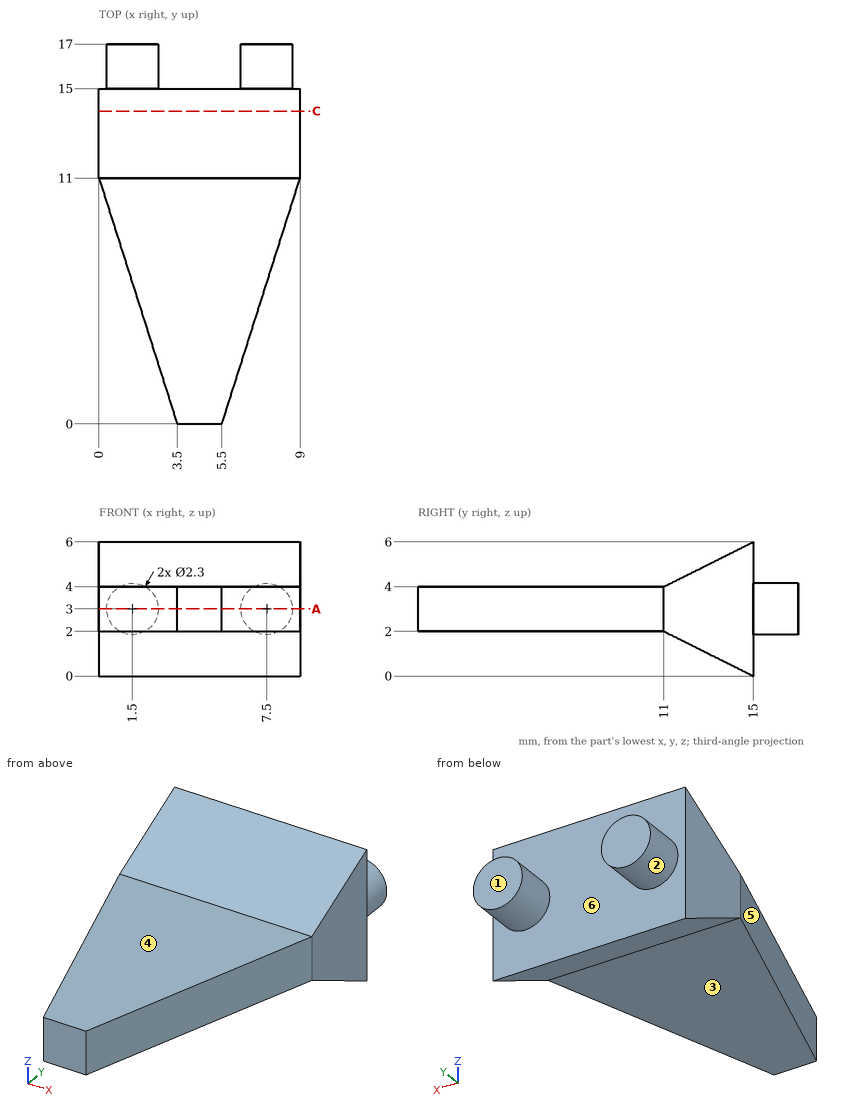
Study the drawing (mm; zero at the part's minimum x, y, z) and answer. A direction names the side the tool comes from. Round coordinates to 2 decimals unless told otherwise and drop trailing zeros. Order: outer loops, then holes, each group sorted by start corner. A loop starts at its lowest first (then second) coordinate and runs counter-clockwise, first axis right, second up. Notation, with made-up numbers: (6.25, 36.25) -> (18.25, 36.25) arc R28 ccw to (18.25, 69.25) -> close; hole circle Ø9 at (77.25, 88). An arc over 180 degrees is marked (long way). Answer as CSV lines item,"result". Start each with the question number.
(1) A tool of negligible diameter and unlimited length cuts with its end or side. For the marked faces 1, 2 and 3, from which of +Z, -Z, +X, -X, +Y, -Y can it reach the whole face along a straight path? Write none if from no direction.
(2) The part is cut by section C-C (y = 14). Determine the outline of the cut face in (x, z), then the cut area to 3 significant figures.
(3) A flat-ended cylindrical pin translates along its axis: pin 1 Ø4.5 at (x, y) = (5.5, 5.5) entering from -Z. Find the tip coordinate at first contact, or state that the pin passes through.
(4) For a pull along X with two mould halves and no side action, classify the marked faces 4, 5 and 6 as +X half, -X half, draft (parallel to the pull), parting line (faces both ways), or undercut.
(5) The part is cut by section A-A (z = 3). Determine the outline of the cut face in (x, y).
(6) Find the intervals of material crossed by probe 1 along Z at (x, y) = (8, 8); probe 2 along Y at (x, z) = (5, 2.5); probe 3 along Y at (x, z) = (2, 4.75), in increasing order. Write a range as from..to.
Evaluation:
1,face 1,"+Z, -Z, +X, -X, +Y"
1,face 2,"+Y"
1,face 3,"-Z, +X, -X, -Y"
2,outline,"(0, 0.5) -> (9, 0.5) -> (9, 5.5) -> (0, 5.5) -> close"
2,area,"45.0 mm²"
3,pin 1,"z = 2"
4,face 4,"draft"
4,face 5,"-X half"
4,face 6,"undercut"
5,outline,"(0, 11) -> (3.5, 0) -> (5.5, 0) -> (9, 11) -> (9, 15) -> (8.65, 15) -> (8.65, 17) -> (6.35, 17) -> (6.35, 15) -> (2.65, 15) -> (2.65, 17) -> (0.35, 17) -> (0.35, 15) -> (0, 15) -> close"
6,probe 1,"2..4"
6,probe 2,"0..15"
6,probe 3,"12.5..15"
